Geometry: final body of the model. Coordinates: model frame, mm. Face numbers are marked on the shaded views. A direction names the side the tool comes from. Round coordinates to 2 decimals unless told otherwise and drop trailing zeros. Write each loop counter-clockwise with the first axis right and the second up, starting at its lowest first coordinate (ties: lowest second). Pieces come first, ordered by that corner, then holes. Notation, with made-up numbers: (81.25, -17) - (118.25, -17) arc R8 ccw to (118.25, -11) - close; hole circle Ø8 at (83.25, 28). An arc over 180 degrees is marked (long way). Write each question's results on one line, items separated by ' | '.
from build123d import *
from OCP.BRepFilletAPI import BRepFilletAPI_MakeFillet

# Parameters (mm, degrees)
SKETCH1_R               = 1.75
SKETCH1_R_2             = 1.65
SKETCH1_R_3             = 9.5
BOSS_EXTRUDE1_DEPTH     = 2
CUT_EXTRUDE1_DEPTH      = 41.5
BOSS_EXTRUDE2_DEPTH     = 41.5
SKETCH6_W               = 16.079745626
SKETCH6_H               = 7
BOSS_EXTRUDE3_DEPTH     = 1
FILLET1_R               = 4
FILLET1_R_2             = 1
SKETCH7_R               = 1.75
CUT_EXTRUDE2_DEPTH      = 90.76114137
FILLET2_R               = 0.5
CUT_EXTRUDE3_DEPTH      = 90.76114137
SKETCH9_W               = 8.01
SKETCH9_H               = 13.4
SKETCH9_W_2             = 3.51
SKETCH9_H_2             = 5.4
CUT_EXTRUDE4_DEPTH      = 1.25
SKETCH9_4_W             = 3.51
SKETCH9_4_H             = 5.4
CUT_EXTRUDE5_DEPTH      = 90.76114137
ENL_V_MAT_EXTRU_1_DEPTH = 90.627353526


with BuildPart() as part:
    # Sketch1 → Boss-Extrude1 (new body)
    with BuildSketch(Plane(origin=(0, 0, 0), x_dir=(1, 0, 0), z_dir=(0, 1, 0))):
        with BuildLine():
            Line((-22, 70), (22, 70))
            ThreePointArc((22, 70), (31.924250474, 67.945789429), (40.217580929, 62.120740202))
            Line((40.217580929, 62.120740202), (47.510174455, 54.360946457))
            ThreePointArc((47.510174455, 54.360946457), (51.771291303, 47.94288813), (53.674026321, 40.47775659))
            Line((53.674026321, 40.47775659), (55.75, 15))
            Line((55.75, 15), (55.75, -2))
            Line((55.75, -2), (20.75, -2))
            Line((20.75, -2), (20.75, -35))
            Line((20.75, -35), (55.75, -35))
            Line((55.75, -35), (55.75, -70))
            Line((55.75, -70), (-55.75, -70))
            Line((-55.75, -70), (-55.75, -35))
            Line((-55.75, -35), (-20.75, -35))
            Line((-20.75, -35), (-20.75, -2))
            Line((-20.75, -2), (-55.75, -2))
            Line((-55.75, -2), (-55.75, 15))
            Line((-55.75, 15), (-53.674026321, 40.47775659))
            ThreePointArc((-53.674026321, 40.47775659), (-51.771291303, 47.94288813), (-47.510174455, 54.360946457))
            Line((-47.510174455, 54.360946457), (-40.217580929, 62.120740202))
            ThreePointArc((-40.217580929, 62.120740202), (-31.924250474, 67.945789429), (-22, 70))
        make_face()
        with Locations(Location((-46.25, -65.5, 0), (0, 0, 270))):
            Circle(SKETCH1_R, mode=Mode.SUBTRACT)
        with Locations(Location((46.25, -65.5, 0), (0, 0, 270))):
            Circle(SKETCH1_R, mode=Mode.SUBTRACT)
        with Locations(Location((-24, 65.5, 0), (0, 0, 270))):
            Circle(SKETCH1_R, mode=Mode.SUBTRACT)
        with Locations(Location((24, 65.5, 0), (0, 0, 270))):
            Circle(SKETCH1_R, mode=Mode.SUBTRACT)
        with Locations(Location((-25, -42.5, 0), (0, 0, 270))):
            Circle(SKETCH1_R, mode=Mode.SUBTRACT)
        with Locations(Location((-25, -62.5, 0), (0, 0, 270))):
            Circle(SKETCH1_R, mode=Mode.SUBTRACT)
        with Locations(Location((25, -42.5, 0), (0, 0, 270))):
            Circle(SKETCH1_R, mode=Mode.SUBTRACT)
        with Locations(Location((25, -62.5, 0), (0, 0, 270))):
            Circle(SKETCH1_R, mode=Mode.SUBTRACT)
        with Locations(Location((-14, 40, 0), (0, 0, 270))):
            Circle(SKETCH1_R_2, mode=Mode.SUBTRACT)
        with Locations(Location((14, 40, 0), (0, 0, 270))):
            Circle(SKETCH1_R_2, mode=Mode.SUBTRACT)
        with Locations(Location((0, 40, 0), (0, 0, 270))):
            Circle(SKETCH1_R_3, mode=Mode.SUBTRACT)
    extrude(amount=BOSS_EXTRUDE1_DEPTH)

    # Sketch5 → Cut-Extrude1 (cut)
    with BuildSketch(Plane(origin=(20.75, 0, 0), x_dir=(0, 0, -1), z_dir=(1, 0, 0))):
        with BuildLine():
            Line((-25.100189391, 2), (-11.899810609, 2))
            ThreePointArc((-11.899810609, 2), (-12.585473072, -0.929312414), (-14.5, -3.25))
            Line((-14.5, -3.25), (-22.5, -3.25))
            ThreePointArc((-22.5, -3.25), (-24.414526928, -0.929312414), (-25.100189391, 2))
        make_face()
    extrude(amount=-CUT_EXTRUDE1_DEPTH, mode=Mode.SUBTRACT)


with BuildPart() as cut_extrude1_piece_1:
    # of the separate pieces the step leaves, piece 1, a body of its own (cut_extrude1_pieces)
    add(part.part.solids().sort_by_distance((-22, 0, -70))[0])



with BuildPart() as cut_extrude1_piece_2:
    # of the separate pieces the step leaves, piece 2, a body of its own (cut_extrude1_pieces)
    add(part.part.solids().sort_by_distance((-20.75, 0, 35))[0])

    # Sketch5<3> → Boss-Extrude2 (add)
    with BuildSketch(Plane(origin=(20.75, 0, 0), x_dir=(0, 0, -1), z_dir=(1, 0, 0))):
        with BuildLine():
            Line((-24.789872813, 0), (-26.539872813, 0))
            Line((-26.539872813, 0), (-26.539872813, -5))
            Line((-26.539872813, -5), (-10.460127187, -5))
            Line((-10.460127187, -5), (-10.460127187, 0))
            Line((-10.460127187, 0), (-12.210127187, 0))
            ThreePointArc((-12.210127187, 0), (-13.10453935, -1.801513432), (-14.5, -3.25))
            Line((-14.5, -3.25), (-22.5, -3.25))
            ThreePointArc((-22.5, -3.25), (-23.89546065, -1.801513432), (-24.789872813, 0))
        make_face()
    extrude(amount=-BOSS_EXTRUDE2_DEPTH)


with BuildPart() as cut_extrude1_piece_1_1:
    add(cut_extrude1_piece_1.part)

    add(cut_extrude1_piece_2.part)  # Boss-Extrude3 merges Cut-Extrude1 piece 2
    # Sketch6 → Boss-Extrude3 (add, symmetric)
    with BuildSketch(Plane(origin=(0, 0, 0), x_dir=(0, 0, -1), z_dir=(1, 0, 0))):
        with Locations((-18.5, -1.5)):
            Rectangle(SKETCH6_W, SKETCH6_H)
    extrude(amount=BOSS_EXTRUDE3_DEPTH, both=True)

    # Fillet1
    fillet1_edges_1 = [cut_extrude1_piece_1_1.edges().sort_by_distance(p)[0] for p in [
        (0, 0, 26.539872813),
        (0, 0, 10.460127187),
    ]]
    fillet1_edges_2 = [cut_extrude1_piece_1_1.edges().sort_by_distance(p)[0] for p in [
        (0, -5, 26.539872813),
        (0, -5, 10.460127187),
        (-10.875, 2, 25.100189391),
        (10.875, 2, 25.100189391),
        (10.875, 2, 11.899810609),
        (-10.875, 2, 11.899810609),
    ]]
    fillet1 = BRepFilletAPI_MakeFillet(cut_extrude1_piece_1_1.part.solid().wrapped)
    for e in fillet1_edges_1:
        fillet1.Add(FILLET1_R - 0.0001, e.wrapped)
    for e in fillet1_edges_2:
        fillet1.Add(FILLET1_R_2 - 0.0001, e.wrapped)
    add(Compound.cast(fillet1.Shape()), mode=Mode.REPLACE)  # a hair under: the kernel refuses the full size

    # Sketch7 → Cut-Extrude2 (cut, through all)
    with BuildSketch(Plane(origin=(0, 2, 0), x_dir=(1, 0, 0), z_dir=(0, 1, 0))):
        with Locations(Location((15, -4.64, 0), (0, 0, 270))):
            Circle(SKETCH7_R)
        with Locations(Location((-15, -4.64, 0), (0, 0, 90))):
            Circle(SKETCH7_R)
        with Locations(Location((-15, -32.36, 0), (0, 0, 270))):
            Circle(SKETCH7_R)
        with Locations(Location((15, -32.36, 0), (0, 0, 90))):
            Circle(SKETCH7_R)
    extrude(amount=-CUT_EXTRUDE2_DEPTH, mode=Mode.SUBTRACT)

    # Fillet2
    fillet2_edges = [cut_extrude1_piece_1_1.edges().sort_by_distance(p)[0] for p in [
        (-55.75, 1, 35),
        (55.75, 1, 35),
        (55.75, 1, 2),
        (-55.75, 1, 2),
    ]]
    fillet(fillet2_edges, radius=FILLET2_R)

    # Sketch8 → Cut-Extrude3 (cut, through all)
    with BuildSketch(Plane(origin=(0, 2, 0), x_dir=(1, 0, 0), z_dir=(0, 1, 0))):
        with BuildLine():
            Line((-55.75, -61), (-53.75, -61))
            ThreePointArc((-53.75, -61), (-53.042893219, -61.292893219), (-52.75, -62))
            Line((-52.75, -62), (-52.75, -70))
            Line((-52.75, -70), (-55.75, -70))
            Line((-55.75, -70), (-55.75, -61))
        make_face()
        with BuildLine():
            Line((55.75, -61), (53.75, -61))
            ThreePointArc((53.75, -61), (53.042893219, -61.292893219), (52.75, -62))
            Line((52.75, -62), (52.75, -70))
            Line((52.75, -70), (55.75, -70))
            Line((55.75, -70), (55.75, -61))
        make_face()
    extrude(amount=-CUT_EXTRUDE3_DEPTH, mode=Mode.SUBTRACT)

    # Sketch9 → Cut-Extrude4 (cut)
    # profile 1 of 6: a face of its own
    with BuildSketch(Plane(origin=(0, 2, 0), x_dir=(1, 0, 0), z_dir=(0, 1, 0))):
        with Locations((-21.505, 53.3)):
            Rectangle(SKETCH9_W, SKETCH9_H)
        with Locations((-21.505, 55.3)):
            Rectangle(SKETCH9_W_2, SKETCH9_H_2, mode=Mode.SUBTRACT)
    # profile 2 of 6: a face of its own
    with BuildSketch(Plane(origin=(0, 2, 0), x_dir=(1, 0, 0), z_dir=(0, 1, 0))):
        with Locations((-21.505, 55.3)):
            Rectangle(SKETCH9_W_2, SKETCH9_H_2)
    # profile 3 of 6: a face of its own
    with BuildSketch(Plane(origin=(0, 2, 0), x_dir=(1, 0, 0), z_dir=(0, 1, 0))):
        with Locations((0, 59.8)):
            Rectangle(SKETCH9_W, SKETCH9_H)
        with Locations((0, 61.8)):
            Rectangle(SKETCH9_W_2, SKETCH9_H_2, mode=Mode.SUBTRACT)
    # profile 4 of 6: a face of its own
    with BuildSketch(Plane(origin=(0, 2, 0), x_dir=(1, 0, 0), z_dir=(0, 1, 0))):
        with Locations((0, 61.8)):
            Rectangle(SKETCH9_W_2, SKETCH9_H_2)
    # profile 5 of 6: a face of its own
    with BuildSketch(Plane(origin=(0, 2, 0), x_dir=(1, 0, 0), z_dir=(0, 1, 0))):
        with Locations((21.505, 53.3)):
            Rectangle(SKETCH9_W, SKETCH9_H)
        with Locations((21.505, 55.3)):
            Rectangle(SKETCH9_W_2, SKETCH9_H_2, mode=Mode.SUBTRACT)
    # profile 6 of 6: a face of its own
    with BuildSketch(Plane(origin=(0, 2, 0), x_dir=(1, 0, 0), z_dir=(0, 1, 0))):
        with Locations((21.505, 55.3)):
            Rectangle(SKETCH9_W_2, SKETCH9_H_2)
    extrude(amount=-CUT_EXTRUDE4_DEPTH, mode=Mode.SUBTRACT)

    # Sketch9<4> → Cut-Extrude5 (cut, through all)
    with BuildSketch(Plane(origin=(0, 2, 0), x_dir=(1, 0, 0), z_dir=(0, 1, 0))):
        with Locations((-21.505, 55.3)):
            Rectangle(SKETCH9_4_W, SKETCH9_4_H)
        with Locations((0, 61.8)):
            Rectangle(SKETCH9_4_W, SKETCH9_4_H)
        with Locations((21.505, 55.3)):
            Rectangle(SKETCH9_4_W, SKETCH9_4_H)
    extrude(amount=-CUT_EXTRUDE5_DEPTH, mode=Mode.SUBTRACT)

    # Esquisse1 → Enlèv. mat.-Extru.1 (cut, through all)
    with BuildSketch(Plane.XZ):
        with BuildLine():
            Line((17.25, -62.5), (17.25, -68.5))
            ThreePointArc((17.25, -68.5), (16.5, -69.25), (15.75, -68.5))
            Line((15.75, -68.5), (15.75, -62.5))
            ThreePointArc((15.75, -62.5), (16.5, -61.75), (17.25, -62.5))
        make_face()
        with BuildLine():
            Line((-17.25, -62.5), (-17.25, -68.5))
            ThreePointArc((-17.25, -68.5), (-16.5, -69.25), (-15.75, -68.5))
            Line((-15.75, -68.5), (-15.75, -62.5))
            ThreePointArc((-15.75, -62.5), (-16.5, -61.75), (-17.25, -62.5))
        make_face()
        with BuildLine():
            Line((17.5, -62.5), (17.5, -68.5))
            ThreePointArc((17.5, -68.5), (16.5, -69.5), (15.5, -68.5))
            Line((15.5, -68.5), (15.5, -62.5))
            ThreePointArc((15.5, -62.5), (16.5, -61.5), (17.5, -62.5))
        make_face()
        with BuildLine():
            Line((-17.5, -62.5), (-17.5, -68.5))
            ThreePointArc((-17.5, -68.5), (-16.5, -69.5), (-15.5, -68.5))
            Line((-15.5, -68.5), (-15.5, -62.5))
            ThreePointArc((-15.5, -62.5), (-16.5, -61.5), (-17.5, -62.5))
        make_face()
    extrude(amount=-ENL_V_MAT_EXTRU_1_DEPTH, mode=Mode.SUBTRACT)


solid = cut_extrude1_piece_1_1.part
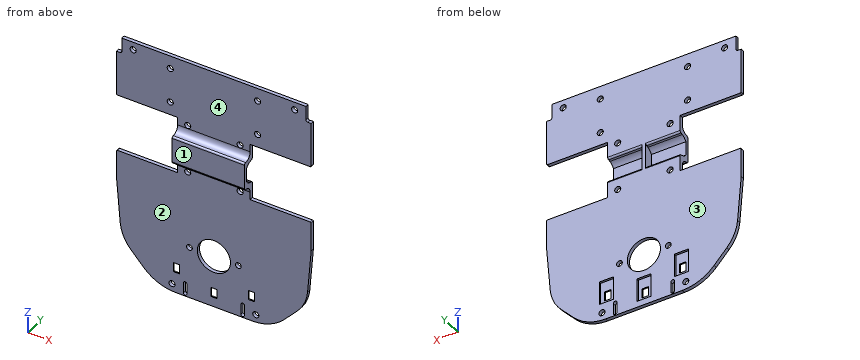
Q1. Section query C-C, the plane z = 42.5. Return loops of the section in (x, y).
Answer block:
outline: (-55.75, 0) - (-26.75, 0) - (-26.75, 2) - (-55.75, 2) - close; (-23.25, 0) - (23.25, 0) - (23.25, 2) - (-23.25, 2) - close; (26.75, 0) - (55.75, 0) - (55.75, 2) - (26.75, 2) - close
Q2. Access query for the marked faces 1 and 2. Directions: +Z, -Z, +X, -X, +Y, -Y. A direction counts if a zero-diameter tool reaches every point of the face in a straight line with its end or side. Return the directions, or none.
Answer block:
face 1: +Z, -Z, +X, -X, -Y | face 2: -Z, +X, -X, -Y
Q3. Section query A-A, the plane z = 4.64. Return loops of the section in (x, y), plus the area to 3 significant figures.
Answer block:
outline: (-20.75, 0) - (-16.75, 0) - (-16.75, 2) - (-20.75, 2) - close; (-13.25, 0) - (13.25, 0) - (13.25, 2) - (-13.25, 2) - close; (16.75, 0) - (20.75, 0) - (20.75, 2) - (16.75, 2) - close | area: 69.0 mm2
Q4. Ray query, line 1 along X through (y, z) = (1.6, 32.36); line 2 along X through (y, z) = (1.05, 42.5); line 3 along X through (y, z) = (1.2, -40). Return the intervals inside material, ascending.
Answer block:
line 1: -20.75 to -16.75, -13.25 to 13.25, 16.75 to 20.75 | line 2: -55.75 to -26.75, -23.25 to 23.25, 26.75 to 55.75 | line 3: -53.71 to -15.65, -12.35 to -9.5, 9.5 to 12.35, 15.65 to 53.71
Q5. Pin query (flat end, axial travel): pin 1 (2 mm diameter, centred on x = -46, y = 1.5, fed in from -Z); pin 2 (1 mm diameter, centred on y = 1.5, z = -66.5, fed in from -X); pin 3 (4 mm diameter, centred on x = 24, z = -65.5, fed in from -Y); pin 4 (5.5 mm diameter, centred on x = -15, z = 4.64, fed in from +Y). Return the tip coordinate at first contact, or that it passes through.
Answer block:
pin 1: z = -57.03 | pin 2: x = -35.56 | pin 3: y = 0 | pin 4: y = 2
Q6. Mould query, pull axis Y, two halves, no side actions, for the marked faces 3 and 4. Classes: pulls with the +Y half, pulls with the -Y half, needs draft (parallel to the pull), parting line crosses it, or undercut.
Answer block:
face 3: pulls with the +Y half | face 4: pulls with the -Y half
Q7. Section query B-B, the plane x = -33. Return loops of the section in (y, z), plus the area to 3 significant figures.
Answer block:
outline: (0, -67.45) - (2, -67.45) - (2, 2) - (0, 2) - close; (0, 35) - (2, 35) - (2, 70) - (0, 70) - close | area: 209 mm2
